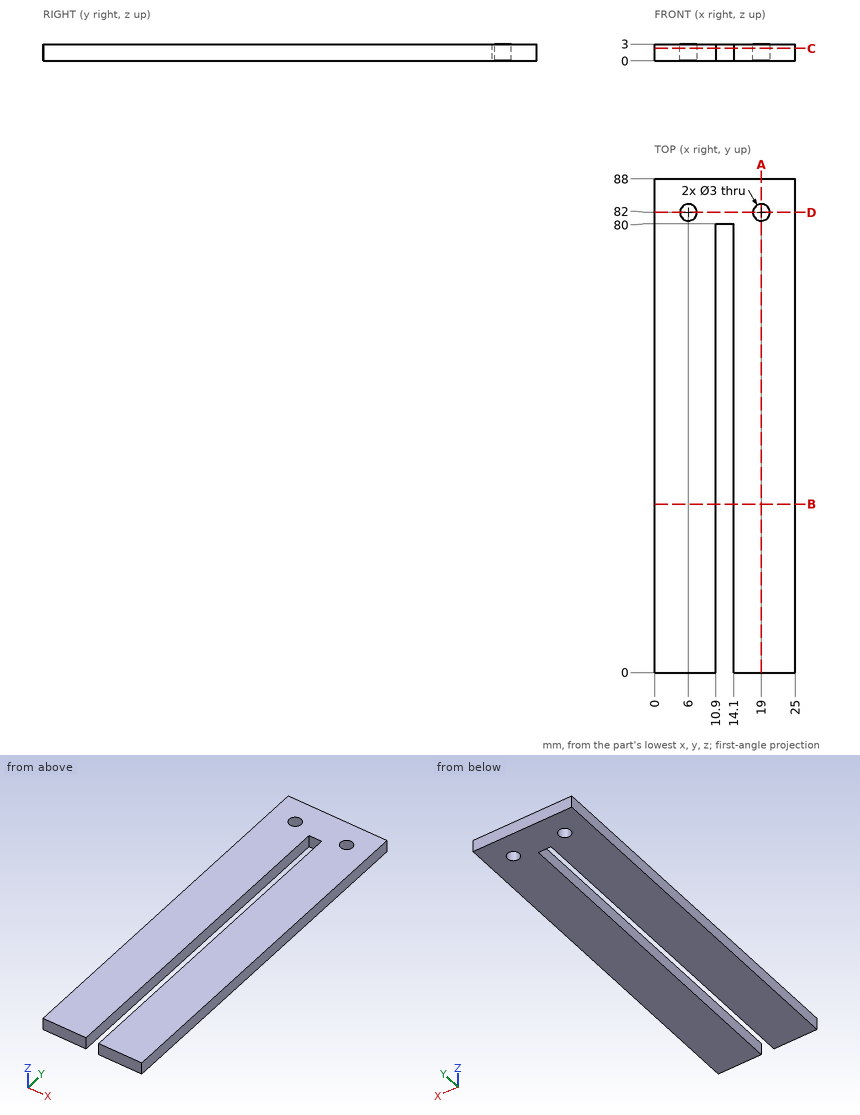
Verification items for this drawing (mm, ordinates from the low corner). Round coordinates to 2 decimals unless told otherwise and drop trailing zeros. Order: outer loops, then holes, each group sorted by start corner. A loop starts at its lowest first (then second) coordinate and runs counter-clockwise, first axis right, second up. Notation, with made-up numbers: M -13,64 L 20,64 A13 ccw 20,88 Z; hole C 80,-27.75 d1. An arc over 180 degrees is marked long. Answer in a Markdown table with one row per item. Add a question column.
Item 1: Sectioned sample at D-D, the plane y = 82. Enter the section's corners in (x, z).
Item 2: Sectioned sample at A-A, the plane x = 19. Enter the section's corners in (y, z).
Item 3: Sectioned sample at B-B, the plane y = 30. Enter the section's corners in (x, z).
Item 4: Sectioned sample at C-C, the plane z = 2.2. Enter the section's corners in (x, y).
Item 5: Depth check by flat-ended pin: pin 1 Ø0.9 at (x, z) = (12.5, 2) entering from -Y. Enter the tip coordinate at first touch or a pass-through.
Item 6: Material ranges on L1, parallel to X at y = 82, z = 1.7; L2, parallel to Y at x = 6, z = 1.8; L3, parallel to X at y = 63, z = 1.3, recorded low to high. Write a range as [from, to].
Filled in:
| question | item | result |
|---|---|---|
| 1 | outline | M 0,0 L 4.5,0 L 4.5,3 L 0,3 Z; M 7.5,0 L 17.5,0 L 17.5,3 L 7.5,3 Z; M 20.5,0 L 25,0 L 25,3 L 20.5,3 Z |
| 2 | outline | M 0,0 L 80.5,0 L 80.5,3 L 0,3 Z; M 83.5,0 L 88,0 L 88,3 L 83.5,3 Z |
| 3 | outline | M 0,0 L 10.9,0 L 10.9,3 L 0,3 Z; M 14.1,0 L 25,0 L 25,3 L 14.1,3 Z |
| 4 | outline | M 0,0 L 10.9,0 L 10.9,80 L 14.1,80 L 14.1,0 L 25,0 L 25,88 L 0,88 Z; hole C 6,82 d3; hole C 19,82 d3 |
| 5 | pin 1 | stops at y = 80 |
| 6 | L1 | x = [0, 4.5], [7.5, 17.5], [20.5, 25] |
| 6 | L2 | y = [0, 80.5], [83.5, 88] |
| 6 | L3 | x = [0, 10.9], [14.1, 25] |
